Geometry: see drawing. Coordinates: mm, zero at the bounding-box minimum. A direction names the side the tool comes from. Give positions to 0.01 mm unless a question says otherwise; leave off trailing zeros. Order: outer loops, then holes, each group sorted by start corner. A loop starts at its lowest first (then second) coordinate and runs counter-clockwise, first axis right, second up. Notation, with made-up numbers: (45.25, -8) - (63.25, -8) arc R18 ccw to (63.25, 25) - close; hole circle Ø9 at (-9, 20). An arc over 180 degrees is marked (long way). One line per item, written item: value.
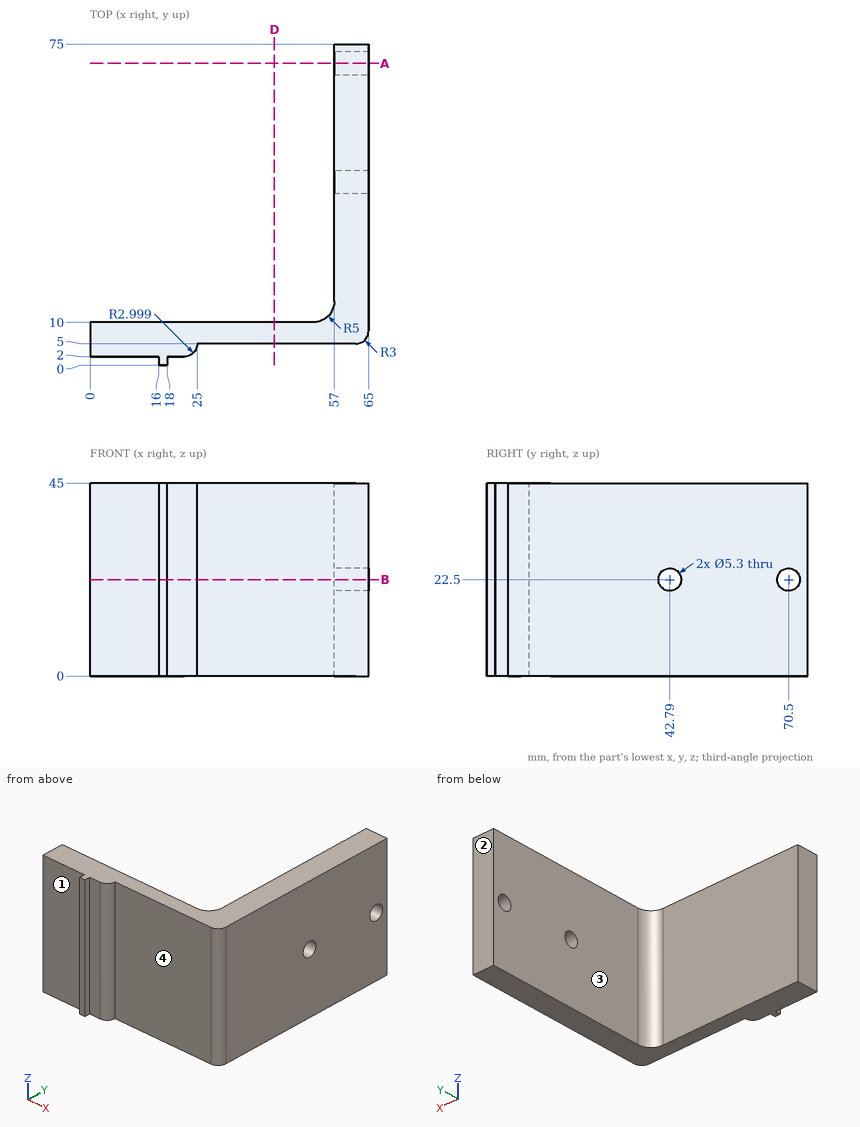
1) Material intervals for line 1 along Y through (x, z) = (62, 22); line 2 along Z through (x, y) = (62.75, 70.5); line 3 along X through (y, z) = (19, 38.5), sorted ascending.
Answers below:
line 1: 5 to 40.19, 45.39 to 67.9, 73.1 to 75
line 2: 0 to 19.85, 25.15 to 45
line 3: 57 to 65
2) Section A-A, the plane y = 70.5. Return loops of the section in (x, z).
Answers below:
outline: (57, 0) - (65, 0) - (65, 19.85) - (57, 19.85) - close; (57, 25.15) - (65, 25.15) - (65, 45) - (57, 45) - close
3) Section D-D, the plane x = 43. Return loops of the section in (y, z).
Answers below:
outline: (5, 0) - (10, 0) - (10, 45) - (5, 45) - close
4) Section B-B, the plane z = 22.5. Count the separate pieces of the cut face and the enclosed holes in it.
Answers below:
separate pieces: 3
enclosed holes: 0
5) First-contact query: pin 1 (1 mm diameter, centred on y = 62.5, z = 7.5, fed in from -X); pin 2 (4 mm diameter, centred on x = 43.5, z = 15, fed in from -Y); pin 3 (1.2 mm diameter, centred on x = 19.5, z = 15, fed in from -Y). Flat tips, straight axial feed; report the tip coordinate or a pass-through.
Answers below:
pin 1: x = 57
pin 2: y = 5
pin 3: y = 2
6) Set-up query: the marked faces 1, 2, 3 and 4. Return all of +Z, -Z, +X, -X, +Y, -Y with unobstructed straight access to the full face (end or side cutting, diameter ignored); none if empty.
Answers below:
face 1: +Z, -Z, -X, -Y
face 2: +Z, -Z, +X, -X, +Y
face 3: +Z, -Z, -X, +Y
face 4: +Z, -Z, +X, -Y
